from build123d import *

# Parameters (mm, degrees)
BOX115_W          = 10
BOX115_H          = 10
BOX115_DEPTH      = 10
CYLINDER017_R     = 4
CYLINDER017_DEPTH = 5
FILLET002_R       = 1
CYLINDER016_R     = 6.25
CYLINDER016_DEPTH = 1.5


with BuildPart() as cube105:
    # Box115 → Box115 (new body)
    with BuildSketch(Plane(origin=(77.4, 9, 0), x_dir=(1, 0, 0), z_dir=(0, 0, 1))):
        with Locations((5, 5)):
            Rectangle(BOX115_W, BOX115_H)
    extrude(amount=BOX115_DEPTH)


with BuildPart() as obj1:
    # Cylinder017 → Cylinder017 (new body)
    with BuildSketch(Plane(origin=(109.54, 14, 6.3), x_dir=(1, 0, 0), z_dir=(0, 0, 1))):
        Circle(CYLINDER017_R)
    extrude(amount=CYLINDER017_DEPTH)

    # Fillet002
    fillet002_edges = [obj1.edges().sort_by_distance(p)[0] for p in [
        (105.54, 14, 11.3),
    ]]
    fillet(fillet002_edges, radius=FILLET002_R)


with BuildPart() as cut071:
    # Cylinder016 → Cylinder016 (new body)
    with BuildSketch(Plane(origin=(109.54, 14, 6.3), x_dir=(1, 0, 0), z_dir=(0, 0, 1))):
        Circle(CYLINDER016_R)
    extrude(amount=CYLINDER016_DEPTH)

    # Fusion016: union obj1
    add(obj1.part)


with BuildPart() as cut071_1:
    # Fusion016 placement: moved
    add(cut071.part.moved(Location((-18, 0, 0))))

    # Cut071: cut Cube105
    add(cube105.part, mode=Mode.SUBTRACT)


solid = cut071_1.part
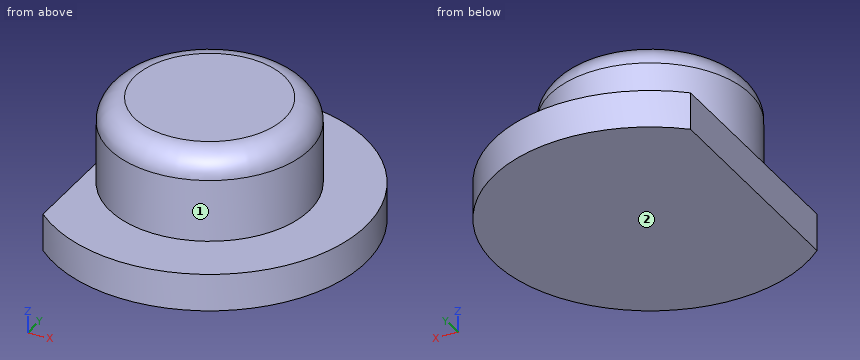
For this review, take the finished solid that the model builds, in its own axes (mm). Face numbers are marked on the shaded views. A direction names the side the tool comes from. Give positions to 0.01 mm unless a question says otherwise; leave off trailing zeros. Write each loop counter-clockwise with the first axis right and the second up, starting at its lowest first coordinate (ties: lowest second). Pieces come first, ordered by that corner, then holes. Notation, with made-up numbers: (-19.5, 48.5) -> (18.5, 48.5) arc R19 ccw to (18.5, 78.5) -> close; hole circle Ø4 at (76, 33). An arc over 180 degrees is marked (long way). Use CSV: the item, a comma, the result in double quotes.
Q1. For P1, Ø3, axis at x = 95, z = 9.5, coming from the -Y side; P2, Ø1.5, axis at x = 95, z = 9, coming from the -Y side; P3, Ø1.5, axis at x = 93.5, z = 9.5, coming from the -Y side, all flat-tipped, find the tip position at first contact; note any pin that passes through.
Conclusion:
P1,"y = 10.51"
P2,"y = 11.06"
P3,"y = 10.19"
Q2. Tool access review of the marked faces 1 and 2: name each direction out of +Z, -Z, +X, -X, +Y, -Y from which nothing blocks a thin tool from reaching the whole face with its end or side.
Conclusion:
face 1,"+Z"
face 2,"-Z, +X, -X, +Y, -Y"
Q3. Take a section at B-B, the plane x = 91.54. Write out the cut boundary in (y, z).
Conclusion:
outline,"(7.75, 6.3) -> (20.25, 6.3) -> (20.25, 7.8) -> (18, 7.8) -> (18, 10.3) arc R1 ccw to (17, 11.3) -> (11, 11.3) arc R1 ccw to (10, 10.3) -> (10, 7.8) -> (7.75, 7.8) -> close"
Q4. To check wall thickness, follow probe 1 along Z at (x, y) = (89.25, 17.75); probe 2 along X at (y, z) = (8.5, 7.3); probe 3 along Y at (x, z) = (91.25, 8.6). State the ranges of each line that lie inside material, in increasing order. Write a range as [from, to].
Conclusion:
probe 1,"[6.3, 7.8]"
probe 2,"[88.57, 94.51]"
probe 3,"[10.01, 17.99]"
Q5. Take a section at A-A, the plane y = 14. Write out the cut boundary in (x, z), then the cut area to 3 significant figures.
Conclusion:
outline,"(87.4, 6.3) -> (97.79, 6.3) -> (97.79, 7.8) -> (95.54, 7.8) -> (95.54, 10.3) arc R1 ccw to (94.54, 11.3) -> (88.54, 11.3) arc R1 ccw to (87.54, 10.3) -> (87.54, 7.8) -> (87.4, 7.8) -> close"
area,"43.2 mm2"
Q6. Take a section at D-D, the plane z = 10.5. Write out the cut boundary in (x, y), then the cut area to 3 significant figures.
Conclusion:
outline,"circle Ø7.96 at (91.54, 14)"
area,"49.8 mm2"
Q7. Take a section at C-C, the plane z = 8.6. Write out the cut boundary in (x, y).
Conclusion:
outline,"circle Ø8 at (91.54, 14)"
